For this review, take the finished solid that the model builds, in its own axes (mm). A direction names the side the tool comes from. Give positions to 0.01 mm unless a question says otherwise; leave off trailing zeros. Loops run counter-clockwise (first coordinate to the right, second up) from the corner with the lowest first, then second, coordinate; pieces in that order, holes last. Notation, with made-up numbers: (6, -24.75) - (16, -24.75) arc R26 cw to (16, 3.25) - close; hole circle Ø5 at (53, 20). An arc over 180 degrees is marked (long way). Answer in a Markdown table with one row per item.
Autodesk Inventor part; units mm, degrees
ref_plane "YZ Plane" through (0, 0, 0) normal (1, 0, 0) x (0, 1, 0)
ref_plane "XZ Plane" through (0, 0, 0) normal (0, 1, 0) x (-1, 0, 0)
ref_plane "XY Plane" through (0, 0, 0) normal (0, 0, 1) x (1, 0, 0)
sketch "Sketch1" plane through (0, 0, 0) normal (0, 1, 0) x (-1, 0, 0)
  line L0 (0, 0) -> (-76.2, 0)
  line L1 (-76.2, 0) -> (-76.2, -76.2)
  line L2 (-76.2, -76.2) -> (0, -76.2)
  line L3 (0, -76.2) -> (0, 0)
  dimension "d0" = 76.2
  dimension "d1" = 76.2
extrude "Extrusion1" add sketch "Sketch1" along normal blind 50.8
sketch "Sketch3" plane through (0, 0, 0) normal (0, -1, 0) x (1, 0, 0)
  line L0 (44.196, -54.102) -> (32.004, -54.102)
  line L1 (32.004, -54.102) -> (32.004, -22.098)
  line L2 (32.004, -22.098) -> (44.196, -22.098)
  line L3 (44.196, -22.098) -> (44.196, -54.102)
  line L4 (76.2, 0) -> (76.2, -76.2)
  line L5 (0, 0) -> (76.2, 0)
  line L6 (32.004, -40.132) -> (6.604, -40.132)
  line L7 (6.604, -40.132) -> (6.604, -36.068)
  line L8 (6.604, -36.068) -> (32.004, -36.068)
  line L9 (32.004, -36.068) -> (32.004, -40.132)
  point P0 (44.196, -38.1)
  point P1 (76.2, -38.1)
  point P2 (38.1, -22.098)
  point P3 (38.1, 0)
  point P4 (6.604, -38.1)
  point P5 (32.004, -38.1)
  dimension "d10" = 32.004
  dimension "d11" = 12.192
  dimension "d12" = 25.4
  dimension "d13" = 4.064
extrude "Extrusion3" add sketch "Sketch3" along normal blind 6.35
sketch "Sketch4" plane through (0, -6.35, 0) normal (0, -1, 0) x (1, 0, 0)
  line L0 (43.942, -49.022) -> (32.258, -49.022)
  line L1 (32.258, -49.022) -> (32.258, -27.178)
  line L2 (32.258, -27.178) -> (43.942, -27.178)
  line L3 (43.942, -27.178) -> (43.942, -49.022)
  line L4 (44.196, -54.102) -> (44.196, -22.098)
  line L5 (32.004, -54.102) -> (44.196, -54.102)
  point P0 (0, 0)
  point P1 (32.258, -38.1)
  point P2 (44.196, -38.1)
  point P3 (38.1, -49.022)
  point P4 (38.1, -54.102)
  dimension "d16" = 21.844
  dimension "d17" = 11.684
extrude "Extrusion4" add sketch "Sketch4" along normal blind 12.7
fillet "Fillet1" radius 25.4 4 edges at (0, 25.4, -76.2) (0, 25.4, 0) (76.2, 25.4, -76.2) (76.2, 25.4, 0)
sketch "Sketch5" plane through (0, 50.8, 0) normal (0, 1, 0) x (1, 0, 0)
  arc A0 (50.8, 0) -> (76.2, 25.4) centre (50.8, 25.4) ccw
  line L0 (76.2, 25.4) -> (76.2, 50.8)
  arc A1 (76.2, 50.8) -> (50.8, 76.2) centre (50.8, 50.8) ccw
  line L1 (50.8, 76.2) -> (25.4, 76.2)
  arc A2 (25.4, 76.2) -> (0, 50.8) centre (25.4, 50.8) ccw
  line L2 (0, 50.8) -> (0, 25.4)
  arc A3 (0, 25.4) -> (25.4, 0) centre (25.4, 25.4) ccw
  line L3 (25.4, 0) -> (50.8, 0)
  arc A4 (25.4, 71.12) -> (5.08, 50.8) centre (25.4, 50.8) ccw
  line L4 (25.4, 71.12) -> (50.8, 71.12)
  arc A5 (71.12, 50.8) -> (50.8, 71.12) centre (50.8, 50.8) ccw
  line L5 (71.12, 50.8) -> (71.12, 25.4)
  arc A6 (50.8, 5.08) -> (71.12, 25.4) centre (50.8, 25.4) ccw
  line L6 (50.8, 5.08) -> (25.4, 5.08)
  arc A7 (5.08, 25.4) -> (25.4, 5.08) centre (25.4, 25.4) ccw
  line L7 (5.08, 25.4) -> (5.08, 50.8)
  point P0 (0, 0)
  point P1 (38.1, 76.2)
  dimension "d21" = 5.08
extrude "Extrusion5" cut sketch "Sketch5" against normal blind 45.72 contours L4 A5 L5 A6 L6 A7 L7 A4
fillet "Fillet2" radius 3.175 8 edges at (0, 0, -38.1) (7.4395, 0, -7.4395) (38.1, 0, 0) (68.7605, 0, -7.4395) (76.2, 0, -38.1) (68.7605, 0, -68.7605) (38.1, 0, -76.2) (7.4395, 0, -68.7605)
chamfer "Chamfer1" distance 19.05 angle 45 8 edges at (38.1, 5.08, -5.08) (11.0316, 5.08, -11.0316) (5.08, 5.08, -38.1) (11.0316, 5.08, -65.1684) (38.1, 5.08, -71.12) (65.1684, 5.08, -65.1684) (71.12, 5.08, -38.1) (65.1684, 5.08, -11.0316)
sketch "Sketch6" plane through (0, 50.8, -50.8) normal (-1, 0, 0) x (0, 0, 1)
  line L0 (7.2288, -10.0054) -> (18.3794, -10.0054)
  line L1 (18.3794, -10.0054) -> (23.9547, -19.6621)
  line L2 (23.9547, -19.6621) -> (18.3794, -29.3188)
  line L3 (18.3794, -29.3188) -> (7.2288, -29.3188)
  line L4 (7.2288, -29.3188) -> (1.6535, -19.6621)
  line L5 (1.6535, -19.6621) -> (7.2288, -10.0054)
  line L6 (16.7677, -26.5271) -> (20.7312, -19.6621)
  line L7 (20.7312, -19.6621) -> (16.7677, -12.797)
  line L8 (16.7677, -12.797) -> (8.8406, -12.797)
  line L9 (8.8406, -12.797) -> (4.877, -19.6621)
  line L10 (4.877, -19.6621) -> (8.8406, -26.5271)
  line L11 (8.8406, -26.5271) -> (16.7677, -26.5271)
  line L12 (23.9558, -24.0955) -> (23.9558, -35.2397)
  line L13 (23.9558, -35.2397) -> (21.1698, -35.2397)
  line L14 (21.1698, -35.2397) -> (21.1698, -28.9211)
  line L15 (21.1698, -28.9211) -> (23.9558, -24.0955)
  line L16 (18.3837, -42.6806) -> (15.5977, -42.6806)
  line L17 (15.5977, -42.6806) -> (15.5977, -31.5364)
  line L18 (7.2396, -31.5364) -> (7.2396, -42.6806)
  line L19 (7.2396, -42.6806) -> (10.0256, -42.6806)
  line L20 (10.0256, -42.6806) -> (10.0256, -31.5364)
  line L21 (1.6675, -24.1328) -> (1.6675, -35.2397)
  line L22 (1.6675, -35.2397) -> (4.4535, -35.2397)
  line L23 (4.4535, -35.2397) -> (4.4535, -28.9583)
  line L24 (4.4535, -28.9583) -> (1.6675, -24.1328)
  line L25 (14.2047, -45.4666) -> (14.2047, -31.5364)
  line L26 (14.2047, -31.5364) -> (11.4186, -31.5364)
  line L27 (11.4186, -31.5364) -> (11.4186, -45.4666)
  line L28 (11.4186, -45.4666) -> (14.2047, -45.4666)
  line L29 (10.0256, -31.5364) -> (7.2396, -31.5364)
  line L30 (15.5977, -42.6806) -> (14.2047, -42.6806) construction
  line L31 (10.0256, -42.6806) -> (11.4186, -42.6806) construction
  line L32 (18.3837, -42.6806) -> (18.3837, -31.5364)
  line L33 (18.3837, -31.5364) -> (15.5977, -31.5364)
  line L34 (12.8041, -44.5678) -> (12.8041, -1.5402) construction
  line L35 (36.5346, -1.5402) -> (-10.9264, -1.5402)
  point P0 (50.8, -50.8)
  point P1 (12.8041, -19.6621)
  dimension "d28" = 11.1506
  dimension "d29" = 2.7916
  dimension "d30" = 2.2177
  dimension "d31" = 2.2232
  dimension "d32" = 2.786
  dimension "d33" = 2.786
  dimension "d34" = 2.786
  dimension "d35" = 2.786
  dimension "d36" = 2.2177
  dimension "d37" = 11.1441
  dimension "d38" = 11.1441
  dimension "d39" = 13.9302
  dimension "d40" = 2.786
  dimension "d41" = 2.786
  dimension "d42" = 2.786
  dimension "d43" = 1.393
  dimension "d44" = 2.7903
sketch "Sketch7" plane through (25.4, 50.8, 0) normal (0, 0, 1) x (1, 0, 0)
  line L0 (4.3171, -27.8388) -> (1.5311, -23.0133)
  line L1 (1.5311, -23.0133) -> (1.5311, -34.1202)
  line L2 (4.7406, -18.5426) -> (8.7041, -25.4077)
  line L3 (7.0924, -28.1993) -> (1.5171, -18.5426)
  line L4 (12.6677, -47.791) -> (12.6677, -4.9445) construction
  line L5 (8.7041, -11.6775) -> (4.7406, -18.5426)
  line L6 (1.5171, -18.5426) -> (7.0924, -8.8859)
  line L7 (1.5311, -34.1202) -> (4.3171, -34.1202)
  line L8 (4.3171, -34.1202) -> (4.3171, -27.8388)
  line L9 (16.6312, -25.4077) -> (20.5948, -18.5426)
  line L10 (23.8183, -18.5426) -> (18.243, -28.1993)
  line L11 (18.243, -28.1993) -> (7.0924, -28.1993)
  line L12 (7.0924, -8.8859) -> (18.243, -8.8859)
  line L13 (18.243, -8.8859) -> (23.8183, -18.5426)
  line L14 (84.753, -4.9445) -> (-59.4176, -4.9445)
  line L15 (16.6312, -11.6775) -> (8.7041, -11.6775)
  line L16 (8.7041, -25.4077) -> (16.6312, -25.4077)
  line L17 (20.5948, -18.5426) -> (16.6312, -11.6775)
  line L18 (21.0333, -34.1202) -> (21.0333, -27.8016)
  line L19 (21.0333, -27.8016) -> (23.8194, -22.976)
  line L20 (23.8194, -34.1202) -> (21.0333, -34.1202)
  line L21 (23.8194, -22.976) -> (23.8194, -34.1202)
  line L22 (18.2473, -41.5611) -> (15.4613, -41.5611)
  line L23 (15.4613, -41.5611) -> (15.4613, -30.4169)
  line L24 (14.0682, -30.4169) -> (11.2822, -30.4169)
  line L25 (18.2473, -30.4169) -> (15.4613, -30.4169)
  line L26 (9.8892, -30.4169) -> (7.1032, -30.4169)
  line L27 (7.1032, -30.4169) -> (7.1032, -41.5611)
  line L28 (7.1032, -41.5611) -> (9.8892, -41.5611)
  line L29 (18.2473, -41.5611) -> (18.2473, -30.4169)
  line L30 (15.4613, -41.5611) -> (14.0682, -41.5611) construction
  line L31 (9.8892, -41.5611) -> (9.8892, -30.4169)
  line L32 (9.8892, -41.5611) -> (11.2822, -41.5611) construction
  line L33 (14.0682, -44.3471) -> (14.0682, -30.4169)
  line L34 (11.2822, -30.4169) -> (11.2822, -44.3471)
  line L35 (11.2822, -44.3471) -> (14.0682, -44.3471)
  point P0 (-25.4, -50.8)
  point P1 (2.3088, -54.2043)
  point P2 (12.6677, -18.5426)
  dimension "d45" = 11.1506
  dimension "d46" = 2.7916
  dimension "d47" = 2.2177
  dimension "d48" = 2.2232
  dimension "d49" = 2.786
  dimension "d50" = 2.786
  dimension "d51" = 2.786
  dimension "d52" = 2.786
  dimension "d53" = 2.2177
  dimension "d54" = 11.1441
  dimension "d55" = 11.1441
  dimension "d56" = 13.9302
  dimension "d57" = 2.786
  dimension "d58" = 2.786
  dimension "d59" = 2.786
  dimension "d60" = 1.393
  dimension "d61" = 2.7903
extrude "Extrusion6" add sketch "Sketch7" along normal blind 1.27
chamfer "Chamfer2" distance 1.27 angle 45 11 edges at (47.8264, 25.4112, 1.27) (42.2543, 20.3831, 1.27) (38.0752, 20.3831, 1.27) (33.8962, 20.3831, 1.27) (28.3241, 25.3739, 1.27) (32.1224, 28.8249, 1.27) (38.0677, 25.3923, 1.27) (44.013, 28.8249, 1.27) (46.4306, 37.0858, 1.27) (38.0677, 41.9141, 1.27) (29.7047, 37.0858, 1.27)
properties part number "Hand Base"
1. For faces 4 (the face through (44.196, -3, -38)), 5 (the face through (6.604, -3, -38)), 6 (the face through (32.004, -3, -47)), 7 (the face through (29.744, 27.361, 0.626)), 8 (the face through (65.326, 37.652, -65.01)), list the 3-axis set-ups (+Z, -Z, +X, -X, +Y, -Y) from which the entire face can be reached by the end or side of a thin tool; tool diameter is ignored.
Values:
| item | result |
|---|---|
| face 4 | +Z, -Z, +X, -Y |
| face 5 | +Z, -Z, -X, -Y |
| face 6 | -Z, -X, -Y |
| face 7 | +Z |
| face 8 | +Y |
2. Wall thickness on line 1 (X direction, y = 33.5, z = -42); line 2 (Z direction, x = 38, y = -12.5); line 3 (Z direction, x = 34, y = 31): over which ranges is each line inside the solid? List them lowest first. Write a range as [from, to].
Values:
| item | result |
|---|---|
| line 1 | x = [0, 5.08], [71.12, 76.2] |
| line 2 | z = [-49.02, -27.18] |
| line 3 | z = [-76.2, -71.12], [-5.08, 0] |
3. We need section C-C, the plane y = -12. Give the boundary of the cut face in (x, z), and give its area (3 significant figures).
Values:
| item | result |
|---|---|
| outline | (32.26, -49.02) - (43.94, -49.02) - (43.94, -27.18) - (32.26, -27.18) - close |
| area | 255 mm^2 |
4. Mouldability with a two-part tool opening along Y and no side actions: class faces 1 (the face through (19, -3, -36.068)), 2 (the face through (38, 5.08, -38)), 3 (the face through (46.47, 27.5, 0.63)) as released by +Y, released by -Y, zero draft, split by the parting line, or undercut.
Values:
| item | result |
|---|---|
| face 1 | zero draft |
| face 2 | released by +Y |
| face 3 | undercut |
5. We need section B-B, the plane z = -44. Give the boundary of the cut face in (x, y) (3 decimals).
Values:
| item | result |
|---|---|
| outline | (0, 3.175) arc R3.175 ccw to (3.175, 0) - (32.004, 0) - (32.004, -6.35) - (32.258, -6.35) - (32.258, -19.05) - (43.942, -19.05) - (43.942, -6.35) - (44.196, -6.35) - (44.196, 0) - (73.025, 0) arc R3.175 ccw to (76.2, 3.175) - (76.2, 50.8) - (71.12, 50.8) - (71.12, 24.13) - (52.07, 5.08) - (24.13, 5.08) - (5.08, 24.13) - (5.08, 50.8) - (0, 50.8) - close |
6. Clearance check with flat-ended pins moving along their axes: pin 1 (8 mm diameter, centred on y = 21.5, z = -55.5, fed in from -X); pin 2 (0.6 mm diameter, centred on y = 16.5, z = 0.5, fed in from +X); pin 3 (1 mm diameter, centred on x = 50, y = 35, fed in from +Z). State where each tip first meets the part, or that it passes through.
Values:
| item | result |
|---|---|
| pin 1 | stops at x = 0.01 |
| pin 2 | stops at x = 49.22 |
| pin 3 | stops at z = 0 |
7. We need section A-A, the plane y = 7.5. Give the boundary of the cut face in (x, z).
Values:
| item | result |
|---|---|
| outline | (0, -50.8) arc R25.4 ccw to (25.4, -76.2) - (50.8, -76.2) arc R25.4 ccw to (76.2, -50.8) - (76.2, -25.4) arc R25.4 ccw to (50.8, 0) - (39.47, 0) - (39.47, 1.27) - (36.68, 1.27) - (36.68, 0) - (25.4, 0) arc R25.4 ccw to (0, -25.4) - close; hole (21.71, -50.8) arc R3.69 ccw to (25.4, -54.49) - (50.8, -54.49) arc R3.69 ccw to (54.49, -50.8) - (54.49, -25.4) arc R3.69 ccw to (50.8, -21.71) - (25.4, -21.71) arc R3.69 ccw to (21.71, -25.4) - close |
